```python
from build123d import *

# Parameters (mm, degrees)
F0_W     = 76.2
F0_H     = 76.2
F1_DEPTH = 76.2
F3_DEPTH = 76.201
F4_W     = 25.4
F4_H     = 25.4
F5_DEPTH = 12.7
F6_DEPTH = 25.4


with BuildPart() as f1:
    # F0 (on Top) → F1 (new body)
    with BuildSketch(Plane.XY):
        with Locations((38.1, 38.1)):
            Rectangle(F0_W, F0_H)
    extrude(amount=F1_DEPTH)

    # F2 (on face) → F3 (cut, through all)
    with BuildSketch(Plane.XY.offset(76.2)):
        Polygon((41.968848, 13.647208), (62.551527, 34.223165), (49.343027, 60.156776), (20.597046, 55.608672), (16.039553, 26.864179), align=None)
    extrude(amount=-F3_DEPTH, mode=Mode.SUBTRACT)

    # F4 (on face) → F5 (cut)
    with BuildSketch(Plane.XZ):
        with Locations((38.1, 38.1)):
            Rectangle(F4_W, F4_H)
    extrude(amount=-F5_DEPTH, mode=Mode.SUBTRACT)

    # F4 (on face) → F6 (cut)
    with BuildSketch(Plane.XZ):
        with Locations((38.1, 38.1)):
            Rectangle(F4_W, F4_H)
    extrude(amount=-F6_DEPTH, mode=Mode.SUBTRACT)


solid = f1.part
```
The listing builds one solid part. Answer for the finished solid, in the listing's coordinates (mm). A direction names the side the tool comes from. Give positions to 0.01 mm unless a question says otherwise; leave off trailing zeros. Loops run counter-clockwise (first coordinate to the right, second up) from the corner with the lowest first, then second, coordinate; pieces in that order, holes last. Notation, with made-up numbers: (15, 74.5) - (27, 74.5) arc R20 cw to (27, 113.5) - close; hole circle Ø6 at (56, 9.5). An arc over 180 degrees is marked (long way). Answer as CSV lines item,"result". Start each with the question number.
Item 1: The mould has two halves that part along X. Classify faces 1 (the face through (76.2, 38, 38)), 2 (the face through (56.04, 47.01, 38.63)), 3 (the face through (0, 38, 38)): +X half, -X half, draft (parallel to the pull), parting line (faces both ways), or undercut.
Item 2: Find the intervals of material crossed by line 1 (X direction, y = 17.5, z = 36); line 2 (Y direction, x = 54.5, z = 53.5); line 3 (X direction, y = 33.5, z = 18.5), in increasing order. Write a range as from..to.
Item 3: A cutting plane is placed at A-A on y = 10. Determine the outline of the cut face in (x, z).
Item 4: A cutting plane is placed at C-C on x = 47.5. Determine the outline of the cut face in (y, z), then the cut area to 3 significant figures.
Item 5: For faces 4 (the face through (38, 76.2, 38)), 5 (the face through (23.061, 23.285, 38.633)), 6 (the face through (50.8, 11, 38)), determine the directions among +Z, -Z, +X, -X, +Y, -Y from which every point of the face is accessible in a straight line to the end or side of a thin tool.
Item 6: A cutting plane is placed at D-D on z = 37. Determine the outline of the cut face in (x, y), then the cut area to 3 significant figures.
Item 7: A cutting plane is placed at B-B on z = 8. Determine the outline of the cut face in (x, y), then the cut area to 3 significant figures.
Item 8: This flat-tipped pin is pushed along its axis until it touches: pin 1 (1 mm diameter, centred on x = 51.5, y = 24.5, fed in from +Z). Where does it stop, or does it pass through?
Found:
1,face 1,"+X half"
1,face 2,"undercut"
1,face 3,"-X half"
2,line 1,"x = 0..25.4, 50.8..76.2"
2,line 2,"y = 0..26.17, 50.03..76.2"
2,line 3,"x = 0..17.09, 61.83..76.2"
3,outline,"(0, 0) - (76.2, 0) - (76.2, 76.2) - (0, 76.2) - close; hole (25.4, 25.4) - (50.8, 25.4) - (50.8, 50.8) - (25.4, 50.8) - close"
4,outline,"(0, 0) - (19.18, 0) - (19.18, 25.4) - (0, 25.4) - close; (0, 50.8) - (19.18, 50.8) - (19.18, 76.2) - (0, 76.2) - close; (59.87, 0) - (76.2, 0) - (76.2, 76.2) - (59.87, 76.2) - close"
4,area,"2,220 mm^2"
5,face 4,"+Z, -Z, +X, -X, +Y"
5,face 5,"+Z, -Z"
5,face 6,"-Y"
6,outline,"(0, 0) - (25.4, 0) - (25.4, 22.09) - (16.04, 26.86) - (20.6, 55.61) - (49.34, 60.16) - (62.55, 34.22) - (50.8, 22.48) - (50.8, 0) - (76.2, 0) - (76.2, 76.2) - (0, 76.2) - close"
6,area,"3,890 mm^2"
7,outline,"(0, 0) - (76.2, 0) - (76.2, 76.2) - (0, 76.2) - close; hole (16.04, 26.86) - (41.97, 13.65) - (62.55, 34.22) - (49.34, 60.16) - (20.6, 55.61) - close"
7,area,"4,350 mm^2"
8,pin 1,"passes through"
